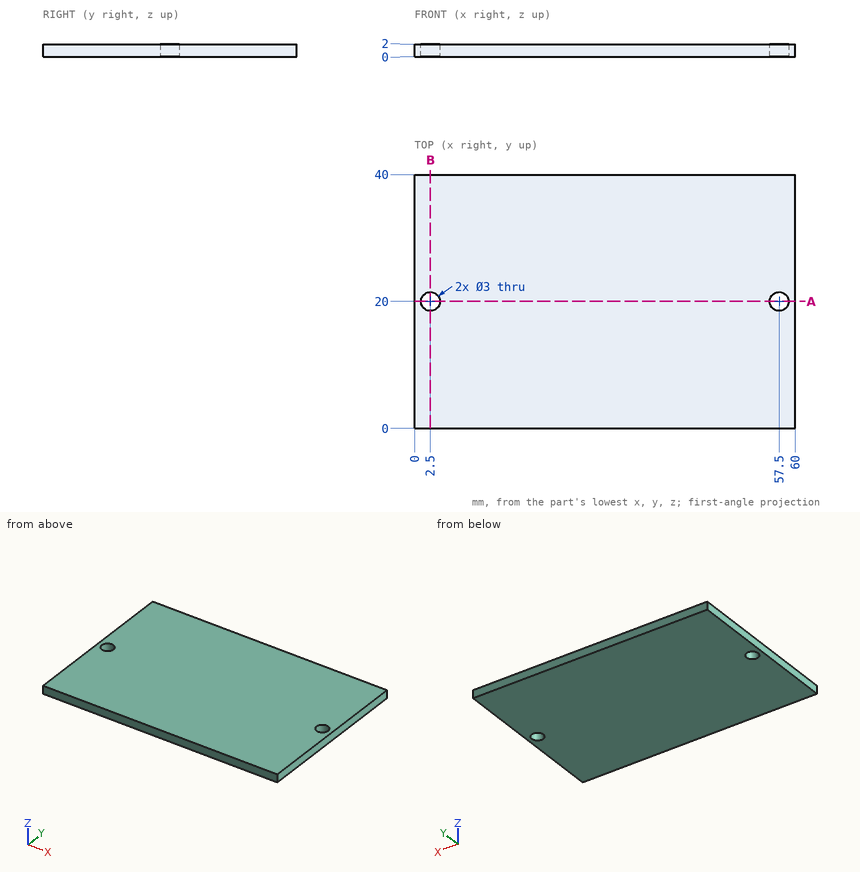
Answer from the drawing. Dimensions are ordinates in mm from the lowest x, y and z of the part. Round coordinates to 2 decimals unless told otherwise and drop trailing zeros. Order: outer loops, then holes, each group sorted by start corner. A loop starts at its lowest first (then second) coordinate and runs counter-clockwise, first axis right, second up.
1) Straight lines are drawn through the part: L1, parallel to Y at x = 2.5, z = 0.9; L2, parallel to X at y = 21, z = 1.05; L3, parallel to Y at x = 3, z = 1.2. For each, find the intervals that lie inside material, in ascending order.
2) The part is cut by section A-A on y = 20. Write down the section's boundary in (x, z), plus the area to 3 significant figures.
3) The part is cut by section B-B on x = 2.5. Write down the section's boundary in (y, z).
Resolved:
1. L1: y = 0 to 18.5, 21.5 to 40
1. L2: x = 0 to 1.38, 3.62 to 56.38, 58.62 to 60
1. L3: y = 0 to 18.59, 21.41 to 40
2. outline: (0, 0) - (1, 0) - (1, 2) - (0, 2) - close; (4, 0) - (56, 0) - (56, 2) - (4, 2) - close; (59, 0) - (60, 0) - (60, 2) - (59, 2) - close
2. area: 108 mm2
3. outline: (0, 0) - (18.5, 0) - (18.5, 2) - (0, 2) - close; (21.5, 0) - (40, 0) - (40, 2) - (21.5, 2) - close
